```python
from build123d import *

# Parameters (mm, degrees)
SKETCH_1_W          = 57
SKETCH_1_H          = 57
SKETCH_1_R          = 2.75
EXTRUDE_1_DEPTH     = 4
SKETCH_2_R          = 27.5
EXTRUDE_2_DEPTH     = 75
SKETCH_3_R          = 19
EXTRUDE_3_DEPTH     = 2
SKETCH_4_R          = 4
EXTRUDE_4_DEPTH     = 23
SKETCH_5_W          = 15
SKETCH_5_H          = 0.5
CUT_EXTRUDE_1_DEPTH = 23


with BuildPart() as part:
    # 草图1 → 凸台-拉伸1 (new body)
    with BuildSketch(Plane.XY):
        with Locations((-6.18683274, 8.316725979)):
            Rectangle(SKETCH_1_W, SKETCH_1_H)
        with Locations((-29.68683274, 31.745551601)):
            Circle(SKETCH_1_R, mode=Mode.SUBTRACT)
        with Locations(Location((17.31316726, 31.745551601, 0), (0, 0, 180))):
            Circle(SKETCH_1_R, mode=Mode.SUBTRACT)
        with Locations((17.31316726, -15.112099644)):
            Circle(SKETCH_1_R, mode=Mode.SUBTRACT)
        with Locations(Location((-29.68683274, -15.112099644, 0), (0, 0, 180))):
            Circle(SKETCH_1_R, mode=Mode.SUBTRACT)
    extrude(amount=EXTRUDE_1_DEPTH)

    # 草图2 → 凸台-拉伸2 (add)
    with BuildSketch(Plane(origin=(0, 0, 0), x_dir=(-1, 0, 0), z_dir=(0, 0, -1))):
        with Locations(Location((6.18683274, 8.316725979, 0), (0, 0, 180))):
            Circle(SKETCH_2_R)
    extrude(amount=EXTRUDE_2_DEPTH)

    # 草图3 → 凸台-拉伸3 (add)
    with BuildSketch(Plane.XY.offset(4)):
        with Locations((-6.18683274, 8.316725979)):
            Circle(SKETCH_3_R)
    extrude(amount=EXTRUDE_3_DEPTH)

    # 草图4 → 凸台-拉伸4 (add)
    with BuildSketch(Plane.XY.offset(6)):
        with Locations((-6.18683274, 8.10325499)):
            Circle(SKETCH_4_R)
    extrude(amount=EXTRUDE_4_DEPTH)

    # 草图5 → 切除-拉伸1 (cut)
    with BuildSketch(Plane(origin=(-2.18683274, 0, 0), x_dir=(0, 0, -1), z_dir=(1, 0, 0))):
        with Locations((-21.5, 11.85325499)):
            Rectangle(SKETCH_5_W, SKETCH_5_H)
    extrude(amount=-CUT_EXTRUDE_1_DEPTH, mode=Mode.SUBTRACT)


solid = part.part
```
Work out the finished part from the listing and answer in its coordinate system (mm). A direction names the side the tool comes from. Give positions to 0.01 mm unless a question says otherwise; leave off trailing zeros. Loops run counter-clockwise (first coordinate to the right, second up) from the corner with the lowest first, then second, coordinate; pieces in that order, holes last. Notation, with made-up numbers: (80, -4) -> (88, -4) arc R19 cw to (88, 28) -> close; hole circle Ø10 at (-28.5, 58.5). An arc over 180 degrees is marked (long way). One line per question, with ' | ' between items. Start each with the question number.
1) Section B-B, the plane y = 0 is taken. Determine the outline of the cut face in (x, z), then the cut area to 3 significant figures.
2) Determine the mould class of faces 1 (the face through (-30.956, -12.672, 1.972)), 2 (the face through (-7.054, 4.198, 17.339)), 3 (the face through (-6, 8, 29)) for opening direction X: +X half, -X half, draft (parallel to the pull), parting line (faces both ways), or undercut.
3) Each of these flat-tipped pins is pushed along its axis until it touches: pin 1 (6 mm diameter, centred on x = 13, z = -49, fed in from +Y); pin 2 (4.5 mm diameter, centred on x = -7, z = 25, fed in from +Y); pin 3 (2 mm diameter, centred on x = -4, z = -59, fed in from +Y). Where does it stop, or does it pass through?
4) Section A-A, the plane x = -31 is taken. Determine the outline of the cut face in (y, z).
5) Straight lines are drawn through the part: L1, parallel to Z at x = -26, y = -0.5; L2, parallel to Z at x = -32, y = 34; L3, parallel to Y at x = -7, z = -35.5. For each, find the intervals that lie inside material, in ascending order.
6) Section D-D, the plane z = 19 is taken. Determine the outline of the cut face in (x, y).
7) Section C-C, the plane x = 8 is taken. Determine the outline of the cut face in (y, z).
8) For faces 4 (the face through (-21.3, -3.2, 5)), 5 (the face through (-34, 8, 0)), 6 (the face through (-7, 8, -75)), 7 (the face through (-7, 36.817, 2)), 8 (the face through (-6, 11.603, 22)), determine the directions among +Z, -Z, +X, -X, +Y, -Y from which every point of the face is accessible in a straight line to the end or side of a thin tool.
Resolved:
1) outline: (-34.69, 0) -> (-32.4, 0) -> (-32.4, -75) -> (20.03, -75) -> (20.03, 0) -> (22.31, 0) -> (22.31, 4) -> (10.9, 4) -> (10.9, 6) -> (-23.27, 6) -> (-23.27, 4) -> (-34.69, 4) -> close | area: 4,230 mm2
2) face 1: undercut | face 2: parting line | face 3: draft
3) pin 1: y = 30.55 | pin 2: y = 11.6 | pin 3: y = 35.79
4) outline: (-20.18, 0) -> (-17.53, 0) -> (-17.53, 4) -> (-20.18, 4) -> close; (-12.7, 0) -> (-3.54, 0) -> (-3.54, -75) -> (20.17, -75) -> (20.17, 0) -> (29.33, 0) -> (29.33, 4) -> (-12.7, 4) -> close; (34.16, 0) -> (36.82, 0) -> (36.82, 4) -> (34.16, 4) -> close
5) L1: -75 to 4 | L2: 0 to 4 | L3: -19.17 to 35.8
6) outline: (-8.12, 11.6) arc R4 ccw (long way) to (-4.25, 11.6) -> close
7) outline: (-20.18, 0) -> (-15.24, 0) -> (-15.24, -75) -> (31.87, -75) -> (31.87, 0) -> (36.82, 0) -> (36.82, 4) -> (20.96, 4) -> (20.96, 6) -> (-4.32, 6) -> (-4.32, 4) -> (-20.18, 4) -> close
8) face 4: +Z | face 5: -Z | face 6: -Z, +X, -X, +Y, -Y | face 7: +Z, -Z, +X, -X, +Y | face 8: +Z, +X, -X, +Y
